```python
from build123d import *

# Parameters (mm, degrees)
BOSS_EXTRUDE1_DEPTH = 3.175
SKETCH2_W           = 304.8
SKETCH2_H           = 3.175
CUT_EXTRUDE1_DEPTH  = 3.175


with BuildPart() as part:
    # Sketch1 → Boss-Extrude1 (new body)
    with BuildSketch(Plane.XY):
        with BuildLine():
            Line((0, 0), (0, -327.025))
            Line((0, -327.025), (349.25, -327.025))
            Line((349.25, -327.025), (349.25, 0))
            ThreePointArc((349.25, 0), (174.625, 174.625), (0, 0))
        make_face()
    extrude(amount=BOSS_EXTRUDE1_DEPTH)

    # Sketch2 → Cut-Extrude1 (cut)
    with BuildSketch(Plane.XY.offset(3.175)):
        with Locations((174.625, -325.4375)):
            Rectangle(SKETCH2_W, SKETCH2_H)
    extrude(amount=-CUT_EXTRUDE1_DEPTH, mode=Mode.SUBTRACT)


solid = part.part
```
Verification items for the finished model (mm, model axes). Coordinates: 2 decimals unless noted, no trailing zeros. Loops run counter-clockwise (first coordinate to the right, second up) from the corner with the lowest first, then second, coordinate; pieces in that order, holes last. Notation, with made-up numbers: (-39.5, 65.25) - (16.5, 65.25) arc R20 ccw to (16.5, 76.25) - close; hole circle Ø4 at (68, -27). An arc over 180 degrees is marked (long way). Answer as a JSON object with one key per item and string values.
(1) Cross-section at B-B, the plane x = 231.5. Record the boundary of the cut face in (y, z) (3 decimals), then the cut area to 3 significant figures.
Response:
{"outline": "(-323.85, 0) - (165.103, 0) - (165.103, 3.175) - (-323.85, 3.175) - close", "area": "1,550 mm²"}
(2) Cross-section at A-A, the plane z = 2.1. Record the boundary of the cut face in (x, y) (3 decimals), then the cut area to 3 significant figures.
Response:
{"outline": "(0, -327.025) - (22.225, -327.025) - (22.225, -323.85) - (327.025, -323.85) - (327.025, -327.025) - (349.25, -327.025) - (349.25, 0) arc R174.625 ccw to (0, 0) - close", "area": "161,000 mm²"}
(3) Cross-section at C-C, the plane y = 77.5. Record the boundary of the cut face in (x, z) (3 decimals), then the cut area to 3 significant figures.
Response:
{"outline": "(18.14, 0) - (331.11, 0) - (331.11, 3.175) - (18.14, 3.175) - close", "area": "994 mm²"}
(4) Scan lines: line 1 along Y through (x, z) = (194, 0.9); line 2 along Y through (x, z) = (159.5, 1.05); line 3 along X through (y, z) = (106.5, 1.5). Record each from-to range of solid material in increasing order.
Response:
{"line 1": "y = -323.85 to 173.55", "line 2": "y = -323.85 to 173.97", "line 3": "x = 36.24 to 313.01"}
